Input: part model. Units: mm. Frame: model coordinates. A direction names the side the tool comes from. Round coordinates to 2 decimals unless told otherwise and drop trailing zeros. Loops run counter-clockwise (first coordinate to the right, second up) from the corner with the lowest first, then second, coordinate; pieces in that order, holes last. Notation, with made-up numbers: M 14.5,-13.75 L 20.5,-13.75 A5 cw 20.5,-8.75 Z; hole C 18,55.25 d9. An arc over 180 degrees is marked long. Return JSON: item names as keys, results as strings. Group by question number.
1) Section B-B (x = 25.4). Output: boundary loops of the cut face in (y, z) (3 decimals), plus the area to 3 significant figures.
2) Material intervals for line 1 (X direction, y = 47, z = 13.75); line 2 (Y direction, x = 19.5, z = 16.5); line 3 (X direction, y = 26, z = 15), sorted ascending. Write a range as from..to.
3) Mould query, pull axis Z, two halves, no side actions, for faces 3 (the face through (25, 39, 0)), 4 (the face through (40.619, 29.507, 7.734)), 5 (the face through (50.8, 38, 9)). Classes: +Z half, -Z half, draft (parallel to the pull), parting line (faces both ways), or undercut.
4) Section D-D (z = 8.75). Output: boundary loops of the cut face in (x, y) (3 decimals).
5) Contact query for flat-ended pins moving along their axis: P1, Ø5, axis at x = 20.62, y = 28.58, coming from the -Z side; P2, Ø1.2, axis at x = 31, y = 28, coming from the +Z side. Output: stop coordinate, or through.
6) Access query for faces 1 (the face through (30, 29, 6.35)), 2 (the face through (25, 0, 9)). Directions: +Z, -Z, +X, -X, +Y, -Y. A direction counts if a zero-diameter tool reaches every point of the face in a straight line with its end or side. Return the directions, or none.
7) Section A-A (y = 44.45). Output: boundary loops of the cut face in (x, z) (3 decimals).
8) Section C-C (z = 17). Output: boundary loops of the cut face in (x, y) (3 decimals).
from build123d import *

# Parameters (mm, degrees)
F0_W     = 50.8
F0_H     = 76.2
F1_DEPTH = 19.05
F2_R     = 3.175
F3_DEPTH = 19.05
F2_R_2   = 2.0193
F4_DEPTH = 12.7
F5_R     = 2.0193
F6_DEPTH = 20.6502


with BuildPart() as f1:
    # F0 (on Top) → F1 (new body)
    with BuildSketch(Plane.XY):
        with Locations((25.4, 38.1)):
            Rectangle(F0_W, F0_H)
    extrude(amount=F1_DEPTH)

    # F2 (on face) → F3 (cut)
    with BuildSketch(Plane.XY.offset(19.05)):
        with Locations((25.4, 44.45)):
            Circle(F2_R)
        with Locations((20.6248, 28.575)):
            Circle(F2_R)
    extrude(amount=-F3_DEPTH, mode=Mode.SUBTRACT)

    # F2 (on face) → F4 (cut)
    with BuildSketch(Plane.XY.offset(19.05)):
        with Locations((25.4, 44.45)):
            Circle(F2_R)
        with Locations((20.6248, 28.575)):
            Circle(F2_R)
        with Locations((30.1498, 28.575)):
            Circle(F2_R_2)
    extrude(amount=-F4_DEPTH, mode=Mode.SUBTRACT)

    # F5 (on face) → F6 (cut)
    with BuildSketch(Plane.YZ.offset(50.8)):
        with Locations((28.575, 9.525)):
            Circle(F5_R)
    extrude(amount=-F6_DEPTH, mode=Mode.SUBTRACT)


solid = f1.part
Returned:
{
 "1": {"outline": "M 0,0 L 41.275,0 L 41.275,19.05 L 0,19.05 Z; M 47.625,0 L 76.2,0 L 76.2,19.05 L 47.625,19.05 Z", "area": "1,330 mm^2"},
 "2": {"line 1": "x = 0..23.51, 27.29..50.8", "line 2": "y = 0..25.61, 31.54..76.2", "line 3": "x = 0..18.77, 22.48..50.8"},
 "3": {"face 3": "-Z half", "face 4": "undercut", "face 5": "draft"},
 "4": {"outline": "M 0,0 L 50.8,0 L 50.8,26.71 L 30.925,26.71 A2.019 cw long 30.925,30.44 L 50.8,30.44 L 50.8,76.2 L 0,76.2 Z; hole C 20.625,28.575 d6.35; hole C 25.4,44.45 d6.35"},
 "5": {"P1": "passes through", "P2": "stops at z = 6.35"},
 "6": {"face 1": "+Z", "face 2": "+Z, -Z, +X, -X, -Y"},
 "7": {"outline": "M 0,0 L 22.225,0 L 22.225,19.05 L 0,19.05 Z; M 28.575,0 L 50.8,0 L 50.8,19.05 L 28.575,19.05 Z"},
 "8": {"outline": "M 0,0 L 50.8,0 L 50.8,76.2 L 0,76.2 Z; hole C 20.625,28.575 d6.35; hole C 25.4,44.45 d6.35; hole C 30.15,28.575 d4.039"}
}
